```python
from build123d import *

# Parameters (mm, degrees)
SKETCH1_W           = 95
SKETCH1_H           = 40
BOSS_EXTRUDE1_DEPTH = 10
SKETCH4_W           = 25
SKETCH4_H           = 15
BOSS_EXTRUDE4_DEPTH = 130
SKETCH5_R           = 5.5
CUT_EXTRUDE1_DEPTH  = 27
SKETCH6_W           = 30
SKETCH6_H           = 6
BOSS_EXTRUDE5_DEPTH = 30
SKETCH7_W           = 30
SKETCH7_H           = 30
BOSS_EXTRUDE6_DEPTH = 8.5


with BuildPart() as part:
    # Sketch1 → Boss-Extrude1 (new body)
    with BuildSketch(Plane(origin=(0, 0, 0), x_dir=(0, 0, -1), z_dir=(1, 0, 0))):
        with Locations((11.585365854, 0.129573171)):
            Rectangle(SKETCH1_W, SKETCH1_H)
    extrude(amount=BOSS_EXTRUDE1_DEPTH)

    # Sketch4 → Boss-Extrude4 (add)
    with BuildSketch(Plane.ZY):
        with Locations((23.414634146, 12.629573171)):
            Rectangle(SKETCH4_W, SKETCH4_H)
        with Locations((23.414634146, -12.370426829)):
            Rectangle(SKETCH4_W, SKETCH4_H)
    extrude(amount=BOSS_EXTRUDE4_DEPTH)

    # Sketch5 → Cut-Extrude1 (cut)
    with BuildSketch(Plane.ZY):
        with Locations((-36.625365854, -2.430426829)):
            Circle(SKETCH5_R)
    extrude(amount=-CUT_EXTRUDE1_DEPTH, mode=Mode.SUBTRACT)

    # Sketch6 → Boss-Extrude5 (add)
    with BuildSketch(Plane(origin=(10, 0, 0), x_dir=(0, 0, -1), z_dir=(1, 0, 0))):
        with Locations((-20.914634146, 0.129573171)):
            Rectangle(SKETCH6_W, SKETCH6_H)
    extrude(amount=BOSS_EXTRUDE5_DEPTH)

    # Sketch7 → Boss-Extrude6 (add)
    with BuildSketch(Plane.XZ.offset(2.870426829)):
        with Locations((25, 20.914634146)):
            Rectangle(SKETCH7_W, SKETCH7_H)
    extrude(amount=BOSS_EXTRUDE6_DEPTH)


solid = part.part
```
Work out the finished part from the listing and answer in its coordinate system (mm). A direction names the side the tool comes from. Give positions to 0.01 mm unless a question says otherwise; leave off trailing zeros. Loops run counter-clockwise (first coordinate to the right, second up) from the corner with the lowest first, then second, coordinate; pieces in that order, holes last. Notation, with made-up numbers: (-19.5, 15) -> (1.5, 15) arc R28 cw to (1.5, 38) -> close; hole circle Ø3 at (-20, -16.5). An arc over 180 degrees is marked (long way). Put each result on its own line as item: value. Start each with the question number.
Item 1: The part is cut by section D-D (y = -16). Give the vertices of the cut face in (x, z).
Item 2: The part is cut by section A-A (x = -33). Give the vertices of the cut face in (y, z).
Item 3: The part is cut by section C-C (z = -33). Give the vertices of the cut face in (x, y).
Item 4: Find the intervals of material crossed by L1, parallel to Y at x = -109, z = 14; L2, parallel to X at y = 5, z = 22; L3, parallel to Y at x = 20, z = 11.5, in increasing order. Write a range as [from, to].
Item 5: Which of the six approach directions +Z, -Z, +X, -X, +Y, -Y give full straight-line access (tool end or side, diameter ignored) to faces 1 (the face through (25, -11.37, 21)), 2 (the face through (-64, -4.87, 23)), 3 (the face through (-64, -12, 10.915))?
Item 6: The part is cut by section B-B (z = 29). Give the vertices of the cut face in (x, y), then the cut area to 4 significant figures.
Item 7: The mould has two halves that part along Z. Classify faces 4 (the face through (-44, -9, 35.915)), 5 (the face through (25, -4, 5.915)), 6 (the face through (-50, -19.87, 17)), 7 (the face through (4.93, -4.537, -31.545)): released by +Z, released by -Z, zero draft, split by the parting line, or undercut.
Item 8: Each of these flat-tipped pins is pushed along its axis until it touches: P1, Ø4.5, axis at x = -78.5, y = 12, coming from the -Z side; P2, Ø6.5, axis at y = -2.43, z = -36.63, coming from the +X side; P3, Ø12, axis at y = -7.5, z = -48.5, coming from the -X side; P4, Ø6, axis at y = 10, z = -11, coming from the +X side. Where does it stop, or does it pass through?
Answers below:
1. outline: (-130, 10.91) -> (0, 10.91) -> (0, -59.09) -> (10, -59.09) -> (10, 35.91) -> (-130, 35.91) -> close
2. outline: (-19.87, 10.91) -> (-4.87, 10.91) -> (-4.87, 35.91) -> (-19.87, 35.91) -> close; (5.13, 10.91) -> (20.13, 10.91) -> (20.13, 35.91) -> (5.13, 35.91) -> close
3. outline: (0, -19.87) -> (10, -19.87) -> (10, -6.57) -> (0, -6.57) -> close; (0, 1.71) -> (10, 1.71) -> (10, 20.13) -> (0, 20.13) -> close
4. L1: [-19.87, -4.87], [5.13, 20.13]
4. L2: [0, 10]
4. L3: [-11.37, 3.13]
5. face 1: +Z, -Z, +X, -Y
5. face 2: +Z, -Z, -X
5. face 3: -Z, -X, +Y, -Y
6. outline: (-130, -19.87) -> (10, -19.87) -> (10, -11.37) -> (40, -11.37) -> (40, 3.13) -> (10, 3.13) -> (10, 20.13) -> (-130, 20.13) -> (-130, 5.13) -> (0, 5.13) -> (0, -4.87) -> (-130, -4.87) -> close
6. area: 4,735 mm2
7. face 4: released by +Z
7. face 5: released by -Z
7. face 6: zero draft
7. face 7: undercut
8. P1: z = 10.91
8. P2: through
8. P3: x = 0
8. P4: x = 10
